For this review, take the finished solid that the model builds, in its own axes (mm). Coordinates: 2 decimals unless noted, no trailing zeros. Loops run counter-clockwise (first coordinate to the right, second up) from the corner with the lowest first, then second, coordinate; pieces in that order, holes last. Notation, with made-up numbers: M 30.25,51 L 58.25,51 A8 cw 58.25,55 Z; hole C 78,67 d11. An arc over 180 degrees is marked long. Use one line per item in the form item = value.
```python
from build123d import *

# Parameters (mm, degrees)
SKETCH1_R           = 2.25
BOSS_EXTRUDE1_DEPTH = 3.175


with BuildPart() as part:
    # Sketch1 → Boss-Extrude1 (new body)
    with BuildSketch(Plane(origin=(0, 0, 0), x_dir=(1, 0, 0), z_dir=(0, 1, 0))):
        Polygon((152.4, 63.5), (152.4, 94.7), (63.5, 94.7), (63.5, 136.7), (25.4, 136.7), (25.4, 133.525), (-25.4, 133.525), (-25.4, 136.7), (-63.5, 136.7), (-63.5, 94.7), (-88.8476, 94.7), (-88.8476, 33.7), (-101.0988, 33.7), (-101.0988, 23.7), (-121.0988, 23.7), (-121.0988, 33.7), (-133.35, 33.7), (-133.35, 94.7), (-152.4, 94.7), (-152.4, 63.5), (-149.225, 63.5), (-149.225, 38.1), (-152.4, 38.1), (-152.4, 12.7), (-149.225, 12.7), (-149.225, -12.7), (-152.4, -12.7), (-152.4, -38.1), (-149.225, -38.1), (-149.225, -63.5), (-152.4, -63.5), (-152.4, -94.7), (-133.35, -94.7), (-133.35, -33.7), (-121.0988, -33.7), (-121.0988, -23.7), (-101.0988, -23.7), (-101.0988, -33.7), (-88.8476, -33.7), (-88.8476, -94.7), (-63.5, -94.7), (-63.5, -136.7), (-25.4, -136.7), (-25.4, -133.525), (25.4, -133.525), (25.4, -136.7), (63.5, -136.7), (63.5, -94.7), (152.4, -94.7), (152.4, -63.5), (149.225, -63.5), (149.225, -38.1), (152.4, -38.1), (152.4, -12.7), (149.225, -12.7), (149.225, 12.7), (152.4, 12.7), (152.4, 38.1), (149.225, 38.1), (149.225, 63.5), align=None)
        with Locations((-140.4411, -86.7)):
            Circle(SKETCH1_R, mode=Mode.SUBTRACT)
        with Locations((-81.7565, -86.7)):
            Circle(SKETCH1_R, mode=Mode.SUBTRACT)
        with Locations((-140.4411, -41.7)):
            Circle(SKETCH1_R, mode=Mode.SUBTRACT)
        with Locations((-81.7565, -41.7)):
            Circle(SKETCH1_R, mode=Mode.SUBTRACT)
        with Locations((-133.35, -12.7)):
            Circle(SKETCH1_R, mode=Mode.SUBTRACT)
        with Locations((81.7565, -86.7)):
            Circle(SKETCH1_R, mode=Mode.SUBTRACT)
        with Locations((140.4411, -86.7)):
            Circle(SKETCH1_R, mode=Mode.SUBTRACT)
        with Locations((81.7565, -41.7)):
            Circle(SKETCH1_R, mode=Mode.SUBTRACT)
        with Locations((140.4411, -41.7)):
            Circle(SKETCH1_R, mode=Mode.SUBTRACT)
        with Locations((133.35, -12.7)):
            Circle(SKETCH1_R, mode=Mode.SUBTRACT)
        with Locations((-133.35, 12.7)):
            Circle(SKETCH1_R, mode=Mode.SUBTRACT)
        with Locations((-111.352954744, 0)):
            Circle(SKETCH1_R, mode=Mode.SUBTRACT)
        with Locations((-140.4411, 41.7)):
            Circle(SKETCH1_R, mode=Mode.SUBTRACT)
        with Locations((-81.7565, 41.7)):
            Circle(SKETCH1_R, mode=Mode.SUBTRACT)
        with Locations((-140.4411, 86.7)):
            Circle(SKETCH1_R, mode=Mode.SUBTRACT)
        with Locations((-81.7565, 86.7)):
            Circle(SKETCH1_R, mode=Mode.SUBTRACT)
        with Locations((111.352954744, 0)):
            Circle(SKETCH1_R, mode=Mode.SUBTRACT)
        with Locations((133.35, 12.7)):
            Circle(SKETCH1_R, mode=Mode.SUBTRACT)
        with Locations((81.7565, 41.7)):
            Circle(SKETCH1_R, mode=Mode.SUBTRACT)
        with Locations((140.4411, 41.7)):
            Circle(SKETCH1_R, mode=Mode.SUBTRACT)
        with Locations((81.7565, 86.7)):
            Circle(SKETCH1_R, mode=Mode.SUBTRACT)
        with Locations((140.4411, 86.7)):
            Circle(SKETCH1_R, mode=Mode.SUBTRACT)
    extrude(amount=BOSS_EXTRUDE1_DEPTH)


solid = part.part
```
1. Consider section C-C on x = -117.5. Write out the cut boundary in (y, z) (3 decimals), plus the area to 3 significant figures.
Computed values:
outline = M 0,-23.7 L 3.175,-23.7 L 3.175,23.7 L 0,23.7 Z
area = 150 mm2
2. Consider section A-A on z = 74. Write out the cut boundary in (x, y) (3 decimals).
Computed values:
outline = M -152.4,0 L -133.35,0 L -133.35,3.175 L -152.4,3.175 Z; M -88.848,0 L 152.4,0 L 152.4,3.175 L -88.848,3.175 Z
3. Consider section B-B on y = 1.4. State how many separate pieces and enclosed holes the cut face has, plus the area to 3 significant figures.
Computed values:
separate_pieces = 1
enclosed_holes = 22
area = 61,400 mm2
4. Consider section D-D on z = 107. Write out the cut boundary in (x, y) (3 decimals).
Computed values:
outline = M -63.5,0 L 63.5,0 L 63.5,3.175 L -63.5,3.175 Z
5. Wall thickness on line 1 along X through (y, z) = (0.8, 41.5) (3 decimals); line 2 along X through (y, z) = (1.5, -86.7); line 3 along X through (y, z) = (2.05, 45.5) (3 decimals): over which ranges is each line inside the solid? List them lowest first. Write a range as from..to.
Computed values:
line_1 = -149.225..-142.682, -138.2..-133.35, -88.848..-83.998, -79.515..79.515, 83.998..138.2, 142.682..149.225
line_2 = -152.4..-142.69, -138.19..-133.35, -88.85..-84.01, -79.51..79.51, 84.01..138.19, 142.69..152.4
line_3 = -149.225..-133.35, -88.848..149.225
6. For pin 1 Ø2.5 at (x, z) = (140.44, 41.7) entering from -Y (3 decimals), flat-tipped, find the tip position at first contact; note if it passes through.
Computed values:
pin_1 = through
